from build123d import *

# Parameters (mm, degrees)
CROQUIS1_R              = 70
SALIENTE_EXTRUIR1_DEPTH = 10
MATRIZC5_COUNT          = 6
CROQUIS9_R              = 27.5
CORTAR_EXTRUIR1_DEPTH   = 10


with BuildPart() as part:
    # Croquis1 → Saliente-Extruir1 (new body)
    with BuildSketch(Plane(origin=(0, 0, 0), x_dir=(0, 0, -1), z_dir=(1, 0, 0))):
        Circle(CROQUIS1_R)
    extrude(amount=SALIENTE_EXTRUIR1_DEPTH)

    # Croquis8 → Taladro roscado M12x1.51 (revolve, cut)
    with BuildSketch(Plane(origin=(10, 60, 0), x_dir=(0, 0, -1), z_dir=(0, 1, 0))):
        Polygon((0, 0), (0, 34.65451825), (5.25, 31.5), (5.25, 0), align=None)
    taladro_roscado_m12x1_51 = revolve(axis=Axis((16.35, 60, 0), (-1, 0, 0)), mode=Mode.SUBTRACT)

    # MatrizC5: Taladro roscado M12x1.51 ×6 about axis
    matrizc5_axis = Axis((0, -0.339409177, 0), (1, 0, 0))
    for i in range(1, MATRIZC5_COUNT):
        add(taladro_roscado_m12x1_51.rotate(matrizc5_axis, i * 360 / MATRIZC5_COUNT), mode=Mode.SUBTRACT)

    # Croquis9 → Cortar-Extruir1 (cut)
    with BuildSketch(Plane(origin=(10, 0, 0), x_dir=(0, 0, -1), z_dir=(1, 0, 0))):
        Circle(CROQUIS9_R)
    extrude(amount=-CORTAR_EXTRUIR1_DEPTH, mode=Mode.SUBTRACT)


solid = part.part
Verification items for the finished model (mm, model axes). Round coordinates to 2 decimals unless told otherwise and drop trailing zeros. Loops run counter-clockwise (first coordinate to the right, second up) from the corner with the lowest first, then second, coordinate; pieces in that order, holes last. Notation, with made-up numbers: (-10.75, -15) - (45.25, -15) arc R25 ccw to (45.25, 22) - close; hole circle Ø6 at (-20, 88). An arc over 180 degrees is marked (long way). Use a Markdown table: item, result. Add a question column.
1. Section check D-D, the plane z = 51.5. Record the boundary of the cut face in (x, y).
2. Release check for a two-part mould opening along Y. For faces 1 (the face through (4.93, -42.594, 55.55)), 2 (the face through (5.07, -25.384, -51.117)), 3 (the face through (0, 1, -30)) record: released by +Y, released by -Y, zero draft, split by the parting line, or undercut.
3. Thickness scan on probe 1 along Y at (x, z) = (4, 0); probe 2 along Y at (x, z) = (6, -54); probe 3 along Z at (x, y) = (2.75, -5). Record the ranges inside material, lowest first. Write a range as [from, to].
4. Section check C-C, the plane x = 2.5. Record the boundary of the cut face in (y, z).
5. Gauge pin test, flat ends, axial feed: pin 1 (1 mm diameter, centred on x = 8, z = 54, fed in from +Y); pin 2 (2 mm diameter, centred on x = 3.5, z = -23.5, fed in from +Y); pin 3 (2 mm diameter, centred on x = 5.5, y = -46.5, fed in from -Z). Record the tip position at first contact, or that the pin passes through.
6. Section check B-B, the plane z = 0. Record the boundary of the cut face in (x, y), plus the area to 3 significant figures.
7. Section check A-A, the plane y = 0. Record the boundary of the cut face in (x, z).
Checks:
| question | item | result |
|---|---|---|
| 1 | outline | (0, -47.41) - (10, -47.41) - (10, -35.7) - (0, -35.7) - close; (0, -25.31) - (10, -25.31) - (10, 24.63) - (0, 24.63) - close; (0, 35.03) - (10, 35.03) - (10, 47.41) - (0, 47.41) - close |
| 2 | face 1 | split by the parting line |
| 2 | face 2 | undercut |
| 2 | face 3 | zero draft |
| 3 | probe 1 | y = [-70, -65.93], [-55.43, -27.5], [27.5, 54.75], [65.25, 70] |
| 3 | probe 2 | y = [-44.54, -35.46], [-25.56, 24.88], [34.78, 44.54] |
| 3 | probe 3 | z = [-69.82, -27.04], [27.04, 69.82] |
| 4 | outline | circle Ø140 at (0, 0); hole circle Ø10.5 at (-60.68, 0); hole circle Ø10.5 at (-30.51, -52.26); hole circle Ø10.5 at (-30.51, 52.26); hole circle Ø55 at (0, 0); hole circle Ø10.5 at (29.83, -52.26); hole circle Ø10.5 at (29.83, 52.26); hole circle Ø10.5 at (60, 0) |
| 5 | pin 1 | stops at y = 45.14 |
| 5 | pin 2 | stops at y = 66.29 |
| 5 | pin 3 | stops at z = -53.2 |
| 6 | outline | (0, -70) - (10, -70) - (10, -65.93) - (0, -65.93) - close; (0, -55.43) - (10, -55.43) - (10, -27.5) - (0, -27.5) - close; (0, 27.5) - (10, 27.5) - (10, 54.75) - (0, 54.75) - close; (0, 65.25) - (10, 65.25) - (10, 70) - (0, 70) - close |
| 6 | area | 640 mm^2 |
| 7 | outline | (0, -70) - (10, -70) - (10, -27.5) - (0, -27.5) - close; (0, 27.5) - (10, 27.5) - (10, 70) - (0, 70) - close |
